Model file for the job. Use its own axes, mm. A direction names the side the tool comes from. Coordinates: 2 decimals unless noted, no trailing zeros. Write each loop counter-clockwise with the first axis right and the second up, starting at its lowest first coordinate (ties: lowest second). Pieces come first, ordered by that corner, then holes. Notation, with made-up numbers: (49, 67) -> (76, 67) arc R28 cw to (76, 94) -> close; hole circle Ø10 at (7.25, 6). An arc over 180 degrees is marked (long way). Write item = value, one per line. Start each with the question number.
Solid Edge part; units mm, degrees
sketch "Sketch1" plane through (0, 0, 0) normal (0, 0, 1) x (1, 0, 0)
  line L0 (-51.7299, 31.1134) -> (-31.7299, 31.1134)
  line L1 (-31.7299, 31.1134) -> (-31.7299, 23.1134)
  line L2 (-31.7299, 23.1134) -> (-51.7299, 23.1134)
  line L3 (-51.7299, 23.1134) -> (-51.7299, 31.1134)
extrude "Protrusion1" add sketch "Sketch1" along normal blind 10
sketch "Sketch2" plane through (-41.7299, 23.1134, 5) normal (0, -1, 0) x (1, 0, 0)
  arc A0 (-10, 5) -> (10, 5) centre (0, -13.3979) cw
extrude "Protrusion2" add sketch "Sketch2" against normal up to vertex (8 mm away) material side at (-41.7299, 23.1134, 12.4921)
shell "Thinwall_1" thickness 0.5 removed faces 1 at (-34.8632, 24.5267, 0)
fillet "Round_1" radius 0.5 8 edges at (-41.7299, 23.1134, 12.5421) (-51.7299, 27.1134, 10) (-51.7299, 23.1134, 5) (-41.7299, 31.1134, 12.5421) (-51.7299, 31.1134, 5) (-31.7299, 31.1134, 5) (-31.7299, 27.1134, 10) (-31.7299, 23.1134, 5)
properties part number "598-205" material "N\\A"
(1) Saw through at B-B (y = 28.5). Give the cut face in (x, z), then the cut area to 3 significant figures.
(2) Mould opens along X. For faces 3 (the face through (-42, 31.113, 6)), 4 (the face through (-51.73, 27, 5)), 5 (the face through (-41.59, 27.06, 12.04)) say: released by +X, released by -X, zero draft, split by the parting line, or undercut.
(3) Saw through at A-A (z = 3). Give the cut face in (x, y), then the cut area to 3 significant figures.
(4) Drop flat-ended pins along their axis: pin 1 Ø3 at (y, z) = (26.5, 10) entering from -X; pin 2 Ø2 at (x, y) = (-42, 26) entering from -Z. Give the stop position or say it passes through.
(5) Drill centre lines: line 1 along Y through (x, z) = (-33.5, 3.5); line 2 along X through (y, z) = (28, 9); line 3 along X through (y, z) = (26.75, 10.25). Where is each one in solid material? Low to high.
(6) 3-axis set-ups, long thin cutter, end or side, ignore diameter. For faces 1 (the face through (-42, 30.613, 6)), 2 (the face through (-31.73, 27, 5)): which of +Z, -Z, +X, -X, +Y, -Y reach the whole face in a straight line?
Returned:
q1.outline = (-51.73, 0) -> (-51.23, 0) -> (-51.23, 9.7) arc R20.44 cw to (-32.23, 9.7) -> (-32.23, 0) -> (-31.73, 0) -> (-31.73, 9.7) arc R0.5 ccw to (-32, 10.14) arc R20.94 ccw to (-51.46, 10.14) arc R0.5 ccw to (-51.73, 9.7) -> close
q1.area = 20.0 mm2
q2.face_3 = zero draft
q2.face_4 = released by -X
q2.face_5 = undercut
q3.outline = (-51.73, 23.61) arc R0.5 ccw to (-51.23, 23.11) -> (-32.23, 23.11) arc R0.5 ccw to (-31.73, 23.61) -> (-31.73, 30.61) arc R0.5 ccw to (-32.23, 31.11) -> (-51.23, 31.11) arc R0.5 ccw to (-51.73, 30.61) -> close; hole (-51.23, 23.61) -> (-32.23, 23.61) -> (-32.23, 30.61) -> (-51.23, 30.61) -> close
q3.area = 26.8 mm2
q4.pin_1 = -51.73
q4.pin_2 = 12
q5.line_1 = 23.11 to 23.61, 30.61 to 31.11
q5.line_2 = -51.73 to -51.23, -32.23 to -31.73
q5.line_3 = -51.26 to -50.1, -33.36 to -32.2
q6.face_1 = -Z
q6.face_2 = +Z, -Z, +X, +Y, -Y
